```python
from build123d import *

# Parameters (mm, degrees)
EXTRUDE_1_DEPTH          = 60
SKETCH_2_W               = 10
SKETCH_2_H               = 40
EXTRUDE_1_2_DEPTH        = 30
SKETCH_3_W               = 40
SKETCH_3_H               = 60
EXTRUDE_2_DEPTH          = 10
CUT_EXTRUDE_1_DEPTH      = 1017.415269464
CUT_EXTRUDE_1_DEPTH_BACK = 1017.415269464
SKETCH_4_W               = 1028.133255753
SKETCH_4_H               = 25
SKETCH_5_W               = 990
SKETCH_5_H               = 10
CUT_EXTRUDE_2_DEPTH      = 16
CUT_EXTRUDE_3_DEPTH      = 1016.775565762
CUT_EXTRUDE_3_DEPTH_BACK = 1016.775565762
SKETCH_7_W               = 20
SKETCH_7_H               = 20


with BuildPart() as part:
    # 草图1 → Extrude 1 (new body)
    with BuildSketch(Plane(origin=(0, 0, 0), x_dir=(1, 0, 0), z_dir=(0, 1, 0))):
        Polygon((0, 10.786516854), (0, 0), (1000, 0), (1000, -20), (0, -20), (0, -30.786516854), (10, -30.786516854), (10, -30), (1010, -30), (1010, 10), (10, 10), (10, 10.786516854), align=None)
    extrude(amount=EXTRUDE_1_DEPTH)

    # 草图2 → Extrude 1 2 (add)
    with BuildSketch(Plane(origin=(0, 60, 0), x_dir=(1, 0, 0), z_dir=(0, 1, 0))):
        with Locations((1005, -10)):
            Rectangle(SKETCH_2_W, SKETCH_2_H)
    extrude(amount=EXTRUDE_1_2_DEPTH)

    # 草图3 → 凸台-拉伸2 (add)
    with BuildSketch(Plane.ZY):
        with Locations((-20, 30)):
            Rectangle(SKETCH_3_W, SKETCH_3_H)
        with Locations((40, 30)):
            Rectangle(SKETCH_3_W, SKETCH_3_H)
    extrude(amount=-EXTRUDE_2_DEPTH)

    # 草图4 → 切除-拉伸1 (cut, two sides: drawn at the far end of the back side and taken through both)
    with BuildSketch(Plane.XY.offset(30).offset(-CUT_EXTRUDE_1_DEPTH_BACK)):
        with Locations((485.933372124, 62.5)):
            Rectangle(SKETCH_4_W, SKETCH_4_H)
    extrude(amount=CUT_EXTRUDE_1_DEPTH + CUT_EXTRUDE_1_DEPTH_BACK, mode=Mode.SUBTRACT)

    # 草图5 → 切除-拉伸2 (cut, symmetric)
    with BuildSketch(Plane.XY.offset(30)):
        with Locations((505, 30)):
            Rectangle(SKETCH_5_W, SKETCH_5_H)
        with Locations((505, 20)):
            Rectangle(SKETCH_5_W, SKETCH_5_H)
    extrude(amount=CUT_EXTRUDE_2_DEPTH, both=True, mode=Mode.SUBTRACT)

    # 草图7 → 切除-拉伸3 (cut, two sides: drawn at the far end of the back side and taken through both)
    with BuildSketch(Plane(origin=(1010, 0, 0), x_dir=(0, 0, -1), z_dir=(1, 0, 0)).offset(-CUT_EXTRUDE_3_DEPTH_BACK)):
        with Locations((-10, 10)):
            Rectangle(SKETCH_7_W, SKETCH_7_H)
    extrude(amount=CUT_EXTRUDE_3_DEPTH + CUT_EXTRUDE_3_DEPTH_BACK, mode=Mode.SUBTRACT)


solid = part.part
```
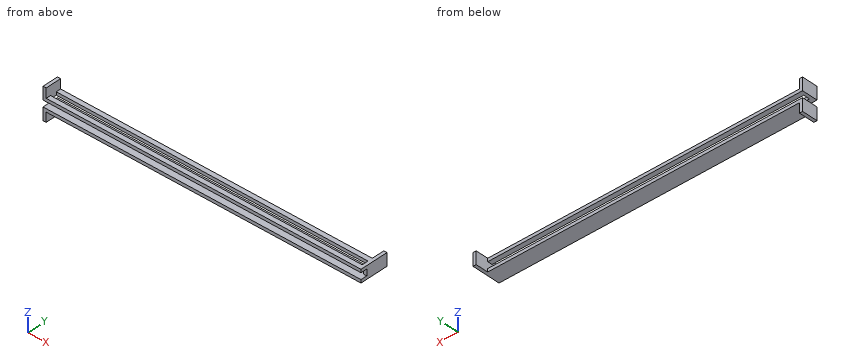
Geometry: final body of the model. Coordinates: model frame, mm. Give positions to 0.01 mm unless a question says otherwise; leave off trailing zeros. Loops run counter-clockwise (first coordinate to the right, second up) from the corner with the lowest first, then second, coordinate; pieces in that order, holes last. Notation, with made-up numbers: (25, 50) - (65, 50) arc R16 ccw to (65, 72) - close; hole circle Ø1 at (-6.75, 10). An arc over 180 degrees is marked (long way). Answer as CSV lines item,"result". Start each with the question number.
(1) Section query A-A (x = 543). Output: boundary loops of the cut face in (y, z), and give its area (3 significant figures).
(2) Section query B-B (y = 81.5). Output: boundary loops of the cut face in (x, z), and give its area (3 significant figures).
(3) Section query C-C (z = 46.5). Output: boundary loops of the cut face in (x, y), and give its area (3 significant figures).
(4) Ray query, line 1 along Z through (x, y) = (478, 5); line 2 along Y through (x, z) = (517.5, 24); line 3 along X through (y, z) = (29, -18.5). Return the intervals inside material, ascending. Write a range as [from, to].
(5) Pin query (flat end, axial travel): P1, Ø10, axis at x = 824.5, y = 33, coming from the +Z side; P2, Ø5, axis at x = 1004.5, z = 11.5, coming from the -Y side; P3, Ø1, axis at y = 29.5, z = 44, coming from the +X side. Return the tip coordinate at first contact, or that it passes through.
Worked answers:
1,outline,"(0, -10) - (50, -10) - (50, 0) - (0, 0) - close; (0, 20) - (15, 20) - (15, 30) - (0, 30) - close; (35, 20) - (50, 20) - (50, 30) - (35, 30) - close"
1,area,"800 mm^2"
2,outline,"(1000, -10) - (1010, -10) - (1010, 30) - (1000, 30) - close"
2,area,"400 mm^2"
3,outline,"(0, 0) - (10, 0) - (10, 50) - (0, 50) - close"
3,area,"500 mm^2"
4,line 1,"z = [-10, 0], [20, 30]"
4,line 2,"y = [0, 15], [35, 50]"
4,line 3,"x = [0, 10]"
5,P1,"stops at z = 30"
5,P2,"stops at y = 20"
5,P3,"stops at x = 10"
